Could you check a few things on this model? Use its own coordinates, in mm. Face numbers are marked on the shaded views. A direction names the side the tool comes from. Round coordinates to 2 decimals unless told otherwise and drop trailing zeros. Order: outer loops, then holes, each group sorted by start corner. A loop starts at its lowest first (then second) coordinate and runs counter-clockwise, first axis right, second up. Notation, with made-up numbers: (80, -24.75) -> (111, -24.75) arc R22 ccw to (111, 13.25) -> close; hole circle Ø9 at (-32.75, 89.25). An arc over 180 degrees is marked (long way). One line per question, with ' | ' between items.
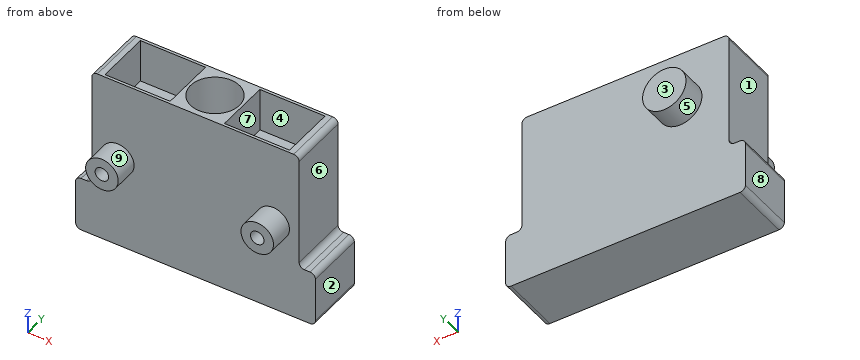
```python
from build123d import *

# Parameters (mm, degrees)
SKETCH_2_W          = 44.15
SKETCH_2_H          = 11
EXTRUDE_1_DEPTH     = 32.2
SKETCH_3_R          = 3
EXTRUDE_2_DEPTH     = 4.5
M3X0_5_1_D          = 2.5
M3X0_5_1_DEPTH      = 5
M3X0_5_1_TIP        = 0.751075774
SKETCH_7_R          = 4
EXTRUDE_3_DEPTH     = 4.5
SKETCH_8_W          = 3
SKETCH_8_H          = 22
CUT_EXTRUDE_1_DEPTH = 16.5
SKETCH_9_W          = 12
SKETCH_9_H          = 10
CUT_EXTRUDE_2_DEPTH = 8
SKETCH_10_R         = 4.5
CUT_EXTRUDE_3_DEPTH = 10
FILLET_1_R          = 1


with BuildPart() as part:
    # 草圖2 → 填料-伸長1 (new body)
    with BuildSketch(Plane.XY):
        Rectangle(SKETCH_2_W, SKETCH_2_H)
    extrude(amount=-EXTRUDE_1_DEPTH)

    # 草圖3 → 填料-伸長2 (add)
    with BuildSketch(Plane.XZ.offset(5.5)):
        with Locations((-14.3, -15.2)):
            Circle(SKETCH_3_R)
        with Locations((14.3, -15.2)):
            Circle(SKETCH_3_R)
    extrude(amount=EXTRUDE_2_DEPTH)

    # M3x0.5  螺絲攻的螺孔鑽1
    with Locations(Plane(origin=(0, -10, 0), x_dir=(-1, 0, 0), z_dir=(0, -1, 0))):
        with Locations((14.3, 15.2), (-14.3, 15.2)):
            Hole(M3X0_5_1_D / 2, depth=M3X0_5_1_DEPTH)
            with Locations((0, 0, -(M3X0_5_1_DEPTH + M3X0_5_1_TIP / 2))):  # 118° drill point
                Cone(0, M3X0_5_1_D / 2, M3X0_5_1_TIP, mode=Mode.SUBTRACT)

    # 草圖7 → 填料-伸長3 (add)
    with BuildSketch(Plane(origin=(0, 5.5, 0), x_dir=(1, 0, 0), z_dir=(0, 1, 0))):
        with Locations((-10.075, 10)):
            Circle(SKETCH_7_R)
    extrude(amount=EXTRUDE_3_DEPTH)

    # 草圖8 → 除料-伸長1 (cut, through all)
    with BuildSketch(Plane(origin=(0, 5.5, 0), x_dir=(1, 0, 0), z_dir=(0, 1, 0))):
        with Locations((-20.575, 11)):
            Rectangle(SKETCH_8_W, SKETCH_8_H)
        with Locations((20.575, 11)):
            Rectangle(SKETCH_8_W, SKETCH_8_H)
    extrude(amount=-CUT_EXTRUDE_1_DEPTH, mode=Mode.SUBTRACT)

    # 草圖9 → 除料-伸長2 (cut)
    with BuildSketch(Plane.XY):
        with Locations((-11, 0)):
            Rectangle(SKETCH_9_W, SKETCH_9_H)
        with Locations((11, 0)):
            Rectangle(SKETCH_9_W, SKETCH_9_H)
    extrude(amount=-CUT_EXTRUDE_2_DEPTH, mode=Mode.SUBTRACT)

    # 草圖10 → 除料-伸長3 (cut)
    with BuildSketch(Plane.XY):
        Circle(SKETCH_10_R)
    extrude(amount=-CUT_EXTRUDE_3_DEPTH, mode=Mode.SUBTRACT)

    # 圓角1
    fillet_1_edges = [part.edges().sort_by_distance(p)[0] for p in [
        (-22.075, 0, -32.2),
        (19.075, 0, 0),
        (-19.075, 0, 0),
        (22.075, 0, -32.2),
        (-22.075, 0, -22),
        (-19.075, 0, -22),
        (22.075, 0, -22),
        (19.075, 0, -22),
    ]]
    fillet(fillet_1_edges, radius=FILLET_1_R)


solid = part.part
```
1. I want a section at C-C on y = 0. List the corners of the cut face in (x, z) for me (3 decimals).
From the geometry:
outline: (-22.075, -31.2) arc R1 ccw to (-21.075, -32.2) -> (21.075, -32.2) arc R1 ccw to (22.075, -31.2) -> (22.075, -23) arc R1 ccw to (21.075, -22) -> (20.075, -22) arc R1 cw to (19.075, -21) -> (19.075, -1) arc R1 ccw to (18.075, 0) -> (17, 0) -> (17, -8) -> (5, -8) -> (5, 0) -> (4.5, 0) -> (4.5, -10) -> (-4.5, -10) -> (-4.5, 0) -> (-5, 0) -> (-5, -8) -> (-17, -8) -> (-17, 0) -> (-18.075, 0) arc R1 ccw to (-19.075, -1) -> (-19.075, -21) arc R1 cw to (-20.075, -22) -> (-21.075, -22) arc R1 ccw to (-22.075, -23) -> close
2. I want a section at A-A on y = -7.5. List the corners of the cut face in (x, z) for me, and give its area (3 significant figures).
From the geometry:
outline: circle Ø6 at (-14.3, -15.2); circle Ø6 at (14.3, -15.2); hole circle Ø2.5 at (-14.3, -15.2); hole circle Ø2.5 at (14.3, -15.2) | area: 46.7 mm²
3. I'm going to push flat-ended pins straight in: pin 1 (1 mm diameter, centred on x = -15.5, z = -28, fed in from -Y); pin 2 (1.5 mm diameter, centred on x = 15, z = -11.5, fed in from +Y); pin 3 (4 mm diameter, centred on y = 2, z = -3, fed in from +X) (3 decimals). Where does each tip first touch, or does it pass through?
From the geometry:
pin 1: stops at y = -5.5 | pin 2: stops at y = 5.5 | pin 3: stops at x = 19.075
4. I want a section at D-D on z = -28. List the corners of the cut face in (x, y) for me (3 decimals).
From the geometry:
outline: (-22.075, -5.5) -> (22.075, -5.5) -> (22.075, 5.5) -> (-22.075, 5.5) -> close
5. I need wall thicknesses on probe 1 along Z at (x, y) = (14.3, -7.4); probe 2 along Y at (x, z) = (10.5, -3.5); probe 3 along X at (y, z) = (1.5, -20) (3 decimals). Which ranges of each line are inside material? Lowest first, please.
From the geometry:
probe 1: z = -18.2 to -16.45, -13.95 to -12.2 | probe 2: y = -5.5 to -5, 5 to 5.5 | probe 3: x = -19.075 to 19.075
6. I want a section at B-B on x = 8.5. List the corners of the cut face in (y, z) for me.
From the geometry:
outline: (-5.5, -32.2) -> (5.5, -32.2) -> (5.5, 0) -> (5, 0) -> (5, -8) -> (-5, -8) -> (-5, 0) -> (-5.5, 0) -> close
7. On a 3-axis mill with a long thin cutter (end or side, diameter ignored), from which of +Z, -Z, +X, -X, +Y, -Y can I reach the whole of each face in a straight line? I mean the marked faces 5, 6, 7, 8 and 9. Say none if no direction works.
From the geometry:
face 5: +Y | face 6: +Z, +X, +Y, -Y | face 7: +Z | face 8: +Z, -Z, -X, +Y, -Y | face 9: -Y
8. If we mould it in two halves opening along X, with no side actions, what happens to the marked faces 1, 2, 3 and 4? For each: pulls with the +X half, pulls with the -X half, needs draft (parallel to the pull), parting line crosses it, or undercut.
From the geometry:
face 1: pulls with the -X half | face 2: pulls with the +X half | face 3: needs draft | face 4: undercut
